Autodesk Inventor part; units mm, degrees
ref_plane "YZ Plane" through (0, 0, 0) normal (1, 0, 0) x (0, 1, 0)
ref_plane "XZ Plane" through (0, 0, 0) normal (0, 1, 0) x (-1, 0, 0)
ref_plane "XY Plane" through (0, 0, 0) normal (0, 0, 1) x (1, 0, 0)
sketch "Sketch1" plane through (0, 0, 0) normal (0, 1, 0) x (-1, 0, 0)
  line L0 (30, 65) -> (-30, 65)
  line L1 (-30, 65) -> (-30, -65)
  line L2 (-30, -65) -> (30, -65)
  line L3 (30, -65) -> (30, 65)
  line L4 (30, 65) -> (-30, -65) construction
  line L5 (-30, 65) -> (30, -65) construction
  line L6 (-17.85, 61) -> (-6.15, 61)
  line L7 (-6.15, 61) -> (-6.15, 55.9)
  line L8 (-6.15, 55.9) -> (-17.85, 55.9)
  line L9 (-17.85, 55.9) -> (-17.85, 61)
  line L10 (-30, 6) -> (-36, 6)
  line L11 (-36, 6) -> (-36, 18)
  line L12 (-36, 18) -> (-30, 18)
  line L13 (-30, 18) -> (-30, 6)
  line L14 (-30, 30) -> (-36, 30)
  line L15 (-36, 30) -> (-36, 42)
  line L16 (-36, 42) -> (-30, 42)
  line L17 (-30, 42) -> (-30, 30)
  line L18 (0, 0) -> (0, 6.5854)
  line L19 (0, 6.5854) -> (0, 0)
  line L20 (0, 0) -> (-5.5856, 0)
  line L21 (17.85, 61) -> (6.15, 61)
  line L22 (6.15, 61) -> (6.15, 55.9)
  line L23 (6.15, 55.9) -> (17.85, 55.9)
  line L24 (17.85, 55.9) -> (17.85, 61)
  line L25 (30, 6) -> (36, 6)
  line L26 (36, 6) -> (36, 18)
  line L27 (36, 18) -> (30, 18)
  line L28 (30, 18) -> (30, 6)
  line L29 (30, 30) -> (36, 30)
  line L30 (36, 30) -> (36, 42)
  line L31 (36, 42) -> (30, 42)
  line L32 (30, 42) -> (30, 30)
  line L33 (-17.85, -61) -> (-6.15, -61)
  line L34 (-6.15, -61) -> (-6.15, -55.9)
  line L35 (-6.15, -55.9) -> (-17.85, -55.9)
  line L36 (-17.85, -55.9) -> (-17.85, -61)
  line L37 (-30, -6) -> (-36, -6)
  line L38 (-36, -6) -> (-36, -18)
  line L39 (-36, -18) -> (-30, -18)
  line L40 (-30, -18) -> (-30, -6)
  line L41 (-30, -30) -> (-36, -30)
  line L42 (-36, -30) -> (-36, -42)
  line L43 (-36, -42) -> (-30, -42)
  line L44 (-30, -42) -> (-30, -30)
  line L45 (6.15, -55.9) -> (17.85, -55.9)
  line L46 (17.85, -61) -> (6.15, -61)
  line L47 (6.15, -61) -> (6.15, -55.9)
  line L48 (17.85, -55.9) -> (17.85, -61)
  line L49 (30, -18) -> (30, -6)
  line L50 (36, -42) -> (30, -42)
  line L51 (36, -30) -> (36, -42)
  line L52 (30, -6) -> (36, -6)
  line L53 (36, -6) -> (36, -18)
  line L54 (30, -42) -> (30, -30)
  line L55 (36, -18) -> (30, -18)
  line L56 (30, -30) -> (36, -30)
  circle A0 centre (-0.15, -58.45) radius 1.125
  circle A1 centre (0, 58.45) radius 1.125
  dimension "d0" = 60
  dimension "d1" = 130
  dimension "d2" = 6
  dimension "d3" = 12
  dimension "d4" = 12
  dimension "d5" = 12
  dimension "d6" = 6
  dimension "d9" = 4
  dimension "d10" = 5.1
  dimension "d13" = 12.3
  dimension "d14" = 11.7
  dimension "d15" = 2.25
  dimension "d16" = 2.25
  dimension "d17" = 6.15
  dimension "d18" = 2.55
  dimension "d19" = 6.3
  dimension "d20" = 2.55
extrude "Extrusion1" add sketch "Sketch1" along normal blind 6
properties part number "case_side" material "Acrylic, Clear"
Can you work these out from the model? Positions are in its coordinate system, mm. A direction names the side the tool comes from. Give positions to 0.01 mm unless a question says otherwise; leave off trailing zeros. Loops run counter-clockwise (first coordinate to the right, second up) from the corner with the lowest first, then second, coordinate; pieces in that order, holes last. Notation, with made-up numbers: (-0.75, -11.75) -> (30.25, -11.75) arc R30 ccw to (30.25, 21.25) -> close; hole circle Ø6 at (81, -2.75). An arc over 180 degrees is marked (long way). Return JSON: item names as keys, results as strings.
Q1. I need wall thicknesses on probe 1 along Z at (x, y) = (-8, 3.55); probe 2 along Z at (x, y) = (0, 2.7) (3 decimals); probe 3 along X at (y, z) = (0.45, 0). Which ranges of each line are inside material? Lowest first, please.
Checks:
{"probe 1": "z = -65 to -61, -55.9 to 55.9, 61 to 65", "probe 2": "z = -65 to -59.565, -57.335 to 57.325, 59.575 to 65", "probe 3": "x = -30 to 30"}
Q2. For pin 1 Ø1.5 at (y, z) = (3.5, 59.5) entering from -X; pin 2 Ø1.8 at (x, y) = (32, 2) entering from -Z; pin 3 Ø1.8 at (x, y) = (-33.5, 4.5) entering from +Z, each with a flat end and sliding along its axis, tell me the tip position at first contact or that it passes through.
Checks:
{"pin 1": "stops at x = -30", "pin 2": "stops at z = -42", "pin 3": "stops at z = 42"}
Q3. On a 3-axis mill with a long thin cutter (end or side, diameter ignored), from which of +Z, -Z, +X, -X, +Y, -Y can I reach the whole of each face in a straight line? I mean faces 1 (the face through (0, 3, 65)), 2 (the face through (-12, 3, -55.9)), 3 (the face through (30, 3, 0)), 4 (the face through (-30, 3, 24)), 5 (the face through (-30, 3, -54)). Say none if no direction works.
Checks:
{"face 1": "+Z, +X, -X, +Y, -Y", "face 2": "+Y, -Y", "face 3": "+X, +Y, -Y", "face 4": "-X, +Y, -Y", "face 5": "-Z, -X, +Y, -Y"}
Q4. I want a section at B-B, the plane z = 26. List the corners of the cut face in (x, y) for me, then the cut area to 3 significant figures.
Checks:
{"outline": "(-30, 0) -> (30, 0) -> (30, 6) -> (-30, 6) -> close", "area": "360 mm2"}
Q5. I want a section at A-A, the plane x = 13. List the corners of the cut face in (y, z) for me, then the cut area to 3 significant figures.
Checks:
{"outline": "(0, -65) -> (6, -65) -> (6, -61) -> (0, -61) -> close; (0, -55.9) -> (6, -55.9) -> (6, 55.9) -> (0, 55.9) -> close; (0, 61) -> (6, 61) -> (6, 65) -> (0, 65) -> close", "area": "719 mm2"}
Q6. I want a section at C-C, the plane y = 4. Count the separate pieces of the cut face and the enclosed holes in it, then the cut area to 3 significant figures.
Checks:
{"separate pieces": "1", "enclosed holes": "6", "area": "8,130 mm2"}
Q7. We'd pull the mould along Z, two halves only. Please class faces 6 (the face through (-33, 3, 18)), 7 (the face through (36, 3, -12)), 8 (the face through (-33, 3, -30)), 9 (the face through (-33, 3, -42)): released by +Z, released by -Z, zero draft, split by the parting line, or undercut.
Checks:
{"face 6": "undercut", "face 7": "zero draft", "face 8": "undercut", "face 9": "released by -Z"}
